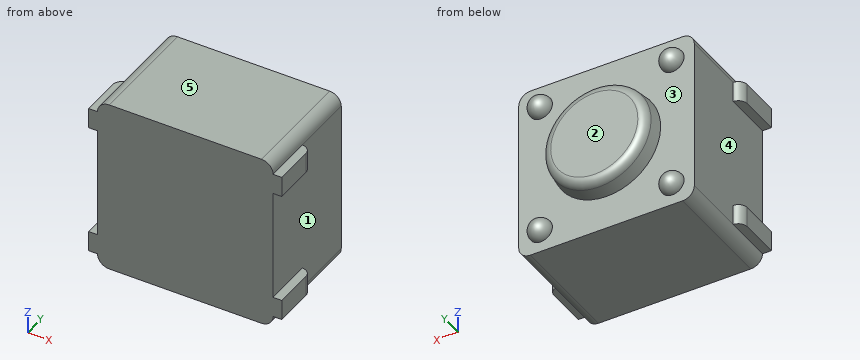
```python
from build123d import *

# Parameters (mm, degrees)
SKETCH1_W               = 6
SKETCH1_H               = 6
BOSS_EXTRUDE1_DEPTH     = 3.9
SKETCH2_W               = 0.7
SKETCH2_H               = 1.674896981
BOSS_EXTRUDE2_DEPTH     = 0.3
SKETCH3_R               = 0.4
BOSS_EXTRUDE3_DEPTH     = 0.4
MIRROR2_COPY_1_SKETCH_W = 0.7
MIRROR2_COPY_1_SKETCH_H = 1.674896981
MIRROR2_COPY_1_DEPTH    = 0.3
MIRROR2_COPY_2_SKETCH_R = 0.4
MIRROR2_COPY_2_DEPTH    = 0.4
FILLET1_R               = 0.4
FILLET2_R               = 0.4
SKETCH4_R               = 1.75
BOSS_EXTRUDE4_DEPTH     = 0.7
DRAFT1_ANGLE            = 8
FILLET3_R               = 0.3
FILLET4_R               = 0.3


with BuildPart() as part:
    # Sketch1 → Boss-Extrude1 (new body)
    with BuildSketch(Plane(origin=(0, 0, 0), x_dir=(1, 0, 0), z_dir=(0, 1, 0))):
        Rectangle(SKETCH1_W, SKETCH1_H)
    extrude(amount=BOSS_EXTRUDE1_DEPTH)

    # Sketch2 → Boss-Extrude2 (add)
    with BuildSketch(Plane(origin=(3, 0, 0), x_dir=(0, 0, -1), z_dir=(1, 0, 0))):
        with Locations((-2.25, 0.837448491)):
            Rectangle(SKETCH2_W, SKETCH2_H)
    boss_extrude2 = extrude(amount=BOSS_EXTRUDE2_DEPTH)

    # Sketch3 → Boss-Extrude3 (add)
    with BuildSketch(Plane(origin=(0, 3.9, 0), x_dir=(1, 0, 0), z_dir=(0, 1, 0))):
        with Locations(Location((2.25, -2.25, 0), (0, 0, 90))):
            Circle(SKETCH3_R)
    boss_extrude3 = extrude(amount=BOSS_EXTRUDE3_DEPTH)

    # Mirror1: Boss-Extrude2, Boss-Extrude3 across plane
    add(boss_extrude2.mirror(Plane.XY))
    add(boss_extrude3.mirror(Plane.XY))

    # Mirror2: Boss-Extrude2, Boss-Extrude3 across plane
    add(boss_extrude2.mirror(Plane(origin=(0, 0, 0), x_dir=(0, 0, 1), z_dir=(1, 0, 0))))
    add(boss_extrude3.mirror(Plane(origin=(0, 0, 0), x_dir=(0, 0, 1), z_dir=(1, 0, 0))))

    # Mirror2 copy 1 sketch → Mirror2 copy 1 (add)
    with BuildSketch(Plane.ZY.offset(3)):
        with Locations((-2.25, 0.837448491)):
            Rectangle(MIRROR2_COPY_1_SKETCH_W, MIRROR2_COPY_1_SKETCH_H)
    extrude(amount=MIRROR2_COPY_1_DEPTH)

    # Mirror2 copy 2 sketch → Mirror2 copy 2 (add)
    with BuildSketch(Plane(origin=(0, 3.9, 0), x_dir=(-1, 0, 0), z_dir=(0, 1, 0))):
        with Locations(Location((2.25, -2.25, 0), (0, 0, 90))):
            Circle(MIRROR2_COPY_2_SKETCH_R)
    extrude(amount=MIRROR2_COPY_2_DEPTH)

    # Fillet1
    fillet1_edges = [part.edges().sort_by_distance(p)[0] for p in [
        (2.25, 4.3, 2.65),
        (2.25, 4.3, -2.65),
        (-2.25, 4.3, -2.65),
        (-2.25, 4.3, 2.65),
    ]]
    fillet(fillet1_edges, radius=FILLET1_R - 0.0001)  # a hair under: the kernel refuses the full size

    # Fillet2
    fillet2_edges = [part.edges().sort_by_distance(p)[0] for p in [
        (3, 1.95, -3),
        (-3, 1.95, -3),
        (-3, 1.95, 3),
        (3, 1.95, 3),
    ]]
    fillet(fillet2_edges, radius=FILLET2_R)

    # Sketch4 → Boss-Extrude4 (add)
    with BuildSketch(Plane(origin=(0, 3.9, 0), x_dir=(1, 0, 0), z_dir=(0, 1, 0))):
        with Locations(Location((0, 0, 0), (0, 0, 90))):
            Circle(SKETCH4_R)
    extrude(amount=BOSS_EXTRUDE4_DEPTH)

    # Draft1
    draft1_faces = [part.faces().sort_by_distance(p)[0] for p in [
        (0, 4.25, 1.75),
    ]]
    draft(draft1_faces, Plane.ZX.offset(4.6), DRAFT1_ANGLE)

    # Fillet3
    fillet3_edges = [part.edges().sort_by_distance(p)[0] for p in [
        (0, 4.6, 1.75),
    ]]
    fillet(fillet3_edges, radius=FILLET3_R)

    # Fillet4
    fillet4_edges = [part.edges().sort_by_distance(p)[0] for p in [
        (-3.3, 1.674896981, -2.25),
        (-3.3, 1.674896981, 2.25),
        (3.3, 1.674896981, -2.25),
        (3.3, 1.674896981, 2.25),
    ]]
    fillet(fillet4_edges, radius=FILLET4_R - 0.0001)  # a hair under: the kernel refuses the full size


solid = part.part
```
For this review, take the finished solid that the model builds, in its own axes (mm). Face numbers are marked on the shaded views. A direction names the side the tool comes from. Round coordinates to 2 decimals unless told otherwise and drop trailing zeros. Order: outer loops, then holes, each group sorted by start corner. A loop starts at its lowest first (then second) coordinate and runs counter-clockwise, first axis right, second up.
Q1. We need section C-C, the plane z = 0. Give the boundary of the cut face in (x, y), plus the area to 3 significant figures.
Findings below:
outline: (-3, 0) - (3, 0) - (3, 3.9) - (1.85, 3.9) - (1.79, 4.34) arc R0.3 ccw to (1.49, 4.6) - (-1.49, 4.6) arc R0.3 ccw to (-1.79, 4.34) - (-1.85, 3.9) - (-3, 3.9) - close
area: 25.9 mm2
Q2. We need section B-B, the plane y = 3.7. Give the boundary of the cut face in (x, z).
Findings below:
outline: (-3, -2.6) arc R0.4 ccw to (-2.6, -3) - (2.6, -3) arc R0.4 ccw to (3, -2.6) - (3, 2.6) arc R0.4 ccw to (2.6, 3) - (-2.6, 3) arc R0.4 ccw to (-3, 2.6) - close
Q3. Mouldability with a two-part tool opening along X and no side actions: class the marked faces 3, 4 and 5 as pulls with the +X half, pulls with the -X half, needs draft (parallel to the pull), parting line crosses it, or undercut.
Findings below:
face 3: undercut
face 4: pulls with the -X half
face 5: needs draft
Q4. Machinability: for the marked faces 1 and 2, which of the approach directions +Z, -Z, +X, -X, +Y, -Y give a long, thin tool a straight path to every point of the face, cutting with its end or side? Answer none if there is none.
Findings below:
face 1: +X, +Y
face 2: +Z, -Z, +X, -X, +Y
Q5. Wall thickness on line 1 (Y direction, x = 2, z = -1.8); line 2 (X direction, y = 2.3, z = -2.3); line 3 (X direction, y = 1.5, z = 2): over which ranges is each line inside the solid? List them lowest first.
Findings below:
line 1: y = 0 to 3.9
line 2: x = -3 to 3
line 3: x = -3.27 to 3.27
Q6. We need section A-A, the plane x = 0. Give the boundary of the cut face in (y, z), plus the area to 3 significant figures.
Findings below:
outline: (0, -3) - (3.9, -3) - (3.9, -1.85) - (4.34, -1.79) arc R0.3 ccw to (4.6, -1.49) - (4.6, 1.49) arc R0.3 ccw to (4.34, 1.79) - (3.9, 1.85) - (3.9, 3) - (0, 3) - close
area: 25.9 mm2
